The listing builds one solid part. Answer for the finished solid, in the listing's coordinates (mm). A direction names the side the tool comes from. Coordinates: 2 decimals unless noted, no trailing zeros. Write each loop counter-clockwise with the first axis right and the second up, starting at its lowest first coordinate (ties: lowest second). Pieces come first, ordered by that corner, then holes.
Autodesk Inventor part; units mm, degrees
ref_plane "YZ Plane" through (0, 0, 0) normal (1, 0, 0) x (0, 1, 0)
ref_plane "XZ Plane" through (0, 0, 0) normal (0, 1, 0) x (-1, 0, 0)
ref_plane "XY Plane" through (0, 0, 0) normal (0, 0, 1) x (1, 0, 0)
sketch "Sketch1" plane through (0, 0, 0) normal (0, 0, 1) x (1, 0, 0)
  line L0 (0, 0) -> (0, 33)
  line L1 (0, 33) -> (40, 33)
  line L2 (40, 33) -> (78.0336, 33)
  line L3 (78.0336, 18) -> (40, 18)
  line L4 (40, 18) -> (40, 0)
  line L5 (40, 0) -> (0, 0)
  circle A0 centre (9.3675, 20) radius 2.5
  circle A1 centre (30, 20) radius 2.5
  circle A2 centre (50.0876, 22) radius 1.75
  circle A3 centre (59.8876, 22) radius 1.75
  line L6 (40, 18) -> (55, 18)
  line L7 (78.0336, 18) -> (78.0336, 33)
  point P0 (0, 16.5)
  dimension "d0" = 40
  dimension "d1" = 33
  dimension "d2" = 5
  dimension "d3" = 5
  dimension "d4" = 10
  dimension "d5" = 10
  dimension "d6" = 20
  dimension "d7" = 20
  dimension "d9" = 3.5
  dimension "d10" = 3.5
  dimension "d11" = 9.8
  dimension "d12" = 4
  dimension "d15" = 15
extrude "Extrusion1" add sketch "Sketch1" along normal blind 2.5
sketch "Sketch3" plane through (0, 0, 2.5) normal (0, 0, 1) x (1, 0, 0)
  point P0 (0, 0)
sketch "Sketch4" plane through (0, 0, 2.5) normal (0, 0, 1) x (1, 0, 0)
  point P0 (0, 0)
equation "\"BendRadius\" = Thickness"
equation "\"BendReliefWidth\" = Thickness"
equation "\"BendReliefDepth\" = 0.5 * Thickness"
equation "\"CornerReliefSize\" = 4 * Thickness"
equation "\"MinimumRemnant\" = 2 * Thickness"
equation "\"TransitionRadius\" = BendRadius"
equation "\"JacobiRadiusSize\" = BendRadius"
equation "\"GapSize\" = Thickness"
Q1. Find the intervals of material crossed by probe 1 along Y at (x, z) = (30, 0.8); probe 2 along Y at (x, z) = (60, 0.4); probe 3 along X at (y, z) = (6.5, 0.8), in increasing order.
Answers below:
probe 1: y = 0 to 17.5, 22.5 to 33
probe 2: y = 18 to 20.25, 23.75 to 33
probe 3: x = 0 to 40
Q2. The part is cut by section C-C, the plane y = 12. Write down the section's boundary in (x, z).
Answers below:
outline: (0, 0) - (40, 0) - (40, 2.5) - (0, 2.5) - close
Q3. The part is cut by section D-D, the plane x = 53.5. Write down the section's boundary in (y, z).
Answers below:
outline: (18, 0) - (33, 0) - (33, 2.5) - (18, 2.5) - close
Q4. Determine the mould class of faces 3 (the face through (0, 16, 1)), 4 (the face through (78.034, 25, 1)), 5 (the face through (38, 33, 1)), 6 (the face through (28.16, 18.31, 1.23)) for opening direction X: released by +X, released by -X, zero draft, split by the parting line, or undercut.
Answers below:
face 3: released by -X
face 4: released by +X
face 5: zero draft
face 6: undercut
Q5. The part is cut by section B-B, the plane z = 1. Write down the section's boundary in (x, y), then the cut area to 3 significant figures.
Answers below:
outline: (0, 0) - (40, 0) - (40, 18) - (78.03, 18) - (78.03, 33) - (0, 33) - close; hole circle Ø5 at (9.37, 20); hole circle Ø5 at (30, 20); hole circle Ø3.5 at (50.09, 22); hole circle Ø3.5 at (59.89, 22)
area: 1,830 mm2
Q6. Which of the six approach directions +Z, -Z, +X, -X, +Y, -Y give full straight-line access (tool end or side, diameter ignored) to faces 1 (the face through (30, 17, 2.5)), 2 (the face through (40, 9, 1))?
Answers below:
face 1: +Z, +X, -X, +Y, -Y
face 2: +Z, -Z, +X, -Y
Q7. Given pin 1 (1 mm diameter, centred on x = 9, y = 21.5, fed in from -Z); pin 2 (1.2 mm diameter, centred on y = 5.5, z = 0.5, fed in from +X); pin 3 (1.5 mm diameter, centred on x = 46.5, y = 21.5, fed in from -Z); pin 4 (1.2 mm diameter, centred on x = 61.5, z = 1, fed in from -Y), each flat-ended and moving along its own axis, determine where each tip first touches the part or whether it passes through.
Answers below:
pin 1: passes through
pin 2: stops at x = 40
pin 3: stops at z = 0
pin 4: stops at y = 18
Q8. The part is cut by section A-A, the plane x = 30. Write down the section's boundary in (y, z).
Answers below:
outline: (0, 0) - (17.5, 0) - (17.5, 2.5) - (0, 2.5) - close; (22.5, 0) - (33, 0) - (33, 2.5) - (22.5, 2.5) - close
